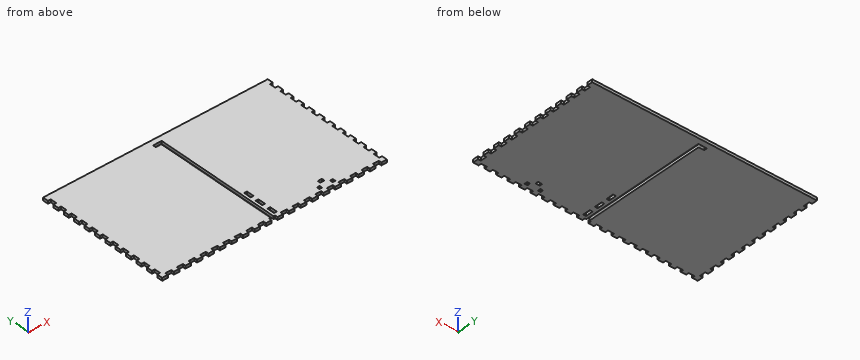
```python
from build123d import *

# Parameters (mm, degrees)
SKETCH1_W           = 508
SKETCH1_H           = 190.5
BOSS_EXTRUDE1_DEPTH = 6.35
SKETCH2_W           = 508
SKETCH2_H           = 190.5
SKETCH2_W_2         = 495.3
SKETCH2_H_2         = 177.8
BOSS_EXTRUDE2_DEPTH = 298.45
SKETCH3_W           = 6.35
SKETCH3_H           = 16.933333333
SKETCH3_H_2         = 16.933333334
CUT_EXTRUDE1_DEPTH  = 12.7
SKETCH4_W           = 6.35
SKETCH4_H           = 15.875
CUT_EXTRUDE2_DEPTH  = 6.35
SKETCH6_W           = 551.127140902
SKETCH6_H           = 227.623239157
CUT_EXTRUDE5_DEPTH  = 305.8
SKETCH5_W           = 13.368421053
SKETCH5_H           = 6.35
SKETCH5_W_2         = 13.368421052
CUT_EXTRUDE6_DEPTH  = 6.35
SKETCH7_W           = 6.35
SKETCH7_H           = 13.854545455
SKETCH7_H_2         = 13.854545454
CUT_EXTRUDE7_DEPTH  = 6.35
SKETCH8_W           = 9.652
SKETCH8_H           = 6.35
SKETCH8_W_2         = 6.35
LEVER_HOLE_DEPTH    = 7.35


with BuildPart() as part:
    # Sketch1 → Boss-Extrude1 (new body)
    with BuildSketch(Plane(origin=(0, 0, 0), x_dir=(1, 0, 0), z_dir=(0, 1, 0))):
        Rectangle(SKETCH1_W, SKETCH1_H)
    extrude(amount=BOSS_EXTRUDE1_DEPTH)

    # Sketch2 → Boss-Extrude2 (add)
    with BuildSketch(Plane(origin=(0, 6.35, 0), x_dir=(1, 0, 0), z_dir=(0, 1, 0))):
        Rectangle(SKETCH2_W, SKETCH2_H)
        Rectangle(SKETCH2_W_2, SKETCH2_H_2, mode=Mode.SUBTRACT)
    extrude(amount=BOSS_EXTRUDE2_DEPTH)

    # Sketch3 → Cut-Extrude1 (cut)
    with BuildSketch(Plane.XY.offset(95.25)):
        with BuildLine():
            Line((-3.302, 283.21), (-3.302, 6.35))
            Line((-3.302, 6.35), (3.302, 6.35))
            Line((3.302, 6.35), (3.302, 292.354))
            Line((3.302, 292.354), (-16.256, 292.354))
            Line((-16.256, 292.354), (-16.256, 285.75))
            Line((-16.256, 285.75), (-5.842, 285.75))
            ThreePointArc((-5.842, 285.75), (-4.045948776, 285.006051224), (-3.302, 283.21))
        make_face()
        with Locations((12.827, 80.433333334)):
            Rectangle(SKETCH3_W, SKETCH3_H)
        with Locations((12.827, 50.8)):
            Rectangle(SKETCH3_W, SKETCH3_H_2)
        with Locations((12.827, 21.166666667)):
            Rectangle(SKETCH3_W, SKETCH3_H)
    extrude(amount=-CUT_EXTRUDE1_DEPTH, mode=Mode.SUBTRACT)

    # Sketch4 → Cut-Extrude2 (cut)
    with BuildSketch(Plane.XY.offset(-88.9)):
        with Locations((-19.431, 284.1625)):
            Rectangle(SKETCH4_W, SKETCH4_H)
        with Locations((-19.431, 255.5875)):
            Rectangle(SKETCH4_W, SKETCH4_H)
        with Locations((-19.431, 227.0125)):
            Rectangle(SKETCH4_W, SKETCH4_H)
        with Locations((-19.431, 198.4375)):
            Rectangle(SKETCH4_W, SKETCH4_H)
        with Locations((-19.431, 169.8625)):
            Rectangle(SKETCH4_W, SKETCH4_H)
        with Locations((-19.431, 141.2875)):
            Rectangle(SKETCH4_W, SKETCH4_H)
        with Locations((-19.431, 112.7125)):
            Rectangle(SKETCH4_W, SKETCH4_H)
        with Locations((-19.431, 84.1375)):
            Rectangle(SKETCH4_W, SKETCH4_H)
        with Locations((-19.431, 55.5625)):
            Rectangle(SKETCH4_W, SKETCH4_H)
        with Locations((-19.431, 26.9875)):
            Rectangle(SKETCH4_W, SKETCH4_H)
    cut_extrude2 = extrude(amount=-CUT_EXTRUDE2_DEPTH, mode=Mode.SUBTRACT)

    # Mirror1: Cut-Extrude2 across plane
    add(cut_extrude2.mirror(Plane.ZY.offset(6.477)), mode=Mode.SUBTRACT)

    # Sketch6 → Cut-Extrude5 (cut, through all)
    with BuildSketch(Plane(origin=(0, 0, 0), x_dir=(1, 0, 0), z_dir=(0, 1, 0))):
        with Locations((15.161260543, 24.911619578)):
            Rectangle(SKETCH6_W, SKETCH6_H)
    extrude(amount=CUT_EXTRUDE5_DEPTH, mode=Mode.SUBTRACT)

    # Sketch5 → Cut-Extrude6 (cut)
    with BuildSketch(Plane(origin=(0, 0, 0), x_dir=(-1, 0, 0), z_dir=(0, -1, 0))):
        with Locations((-234.615789474, -92.075)):
            Rectangle(SKETCH5_W, SKETCH5_H)
        with Locations((-208.547368421, -92.075)):
            Rectangle(SKETCH5_W_2, SKETCH5_H)
        with Locations((-182.478947369, -92.075)):
            Rectangle(SKETCH5_W, SKETCH5_H)
        with Locations((-156.410526316, -92.075)):
            Rectangle(SKETCH5_W, SKETCH5_H)
        with Locations((-130.342105263, -92.075)):
            Rectangle(SKETCH5_W_2, SKETCH5_H)
        with Locations((-104.273684211, -92.075)):
            Rectangle(SKETCH5_W, SKETCH5_H)
        with Locations((-78.205263158, -92.075)):
            Rectangle(SKETCH5_W_2, SKETCH5_H)
        with Locations((-52.136842106, -92.075)):
            Rectangle(SKETCH5_W, SKETCH5_H)
        with Locations((-26.068421052, -92.075)):
            Rectangle(SKETCH5_W, SKETCH5_H)
        with Locations((0, -92.075)):
            Rectangle(SKETCH5_W_2, SKETCH5_H)
        with Locations((26.068421052, -92.075)):
            Rectangle(SKETCH5_W, SKETCH5_H)
        with Locations((52.136842106, -92.075)):
            Rectangle(SKETCH5_W, SKETCH5_H)
        with Locations((78.205263158, -92.075)):
            Rectangle(SKETCH5_W_2, SKETCH5_H)
        with Locations((104.273684211, -92.075)):
            Rectangle(SKETCH5_W, SKETCH5_H)
        with Locations((130.342105263, -92.075)):
            Rectangle(SKETCH5_W_2, SKETCH5_H)
        with Locations((156.410526316, -92.075)):
            Rectangle(SKETCH5_W, SKETCH5_H)
        with Locations((182.478947369, -92.075)):
            Rectangle(SKETCH5_W, SKETCH5_H)
        with Locations((208.547368421, -92.075)):
            Rectangle(SKETCH5_W_2, SKETCH5_H)
        with Locations((234.615789474, -92.075)):
            Rectangle(SKETCH5_W, SKETCH5_H)
    extrude(amount=-CUT_EXTRUDE6_DEPTH, mode=Mode.SUBTRACT)

    # Sketch7 → Cut-Extrude7 (cut)
    with BuildSketch(Plane(origin=(254, 0, 0), x_dir=(0, 0, -1), z_dir=(1, 0, 0))):
        with Locations((-92.075, 285.172727273)):
            Rectangle(SKETCH7_W, SKETCH7_H)
        with Locations((-92.075, 258.618181818)):
            Rectangle(SKETCH7_W, SKETCH7_H_2)
        with Locations((-92.075, 232.063636364)):
            Rectangle(SKETCH7_W, SKETCH7_H)
        with Locations((-92.075, 205.509090909)):
            Rectangle(SKETCH7_W, SKETCH7_H_2)
        with Locations((-92.075, 178.954545455)):
            Rectangle(SKETCH7_W, SKETCH7_H)
        with Locations((-92.075, 152.4)):
            Rectangle(SKETCH7_W, SKETCH7_H_2)
        with Locations((-92.075, 125.845454546)):
            Rectangle(SKETCH7_W, SKETCH7_H)
        with Locations((-92.075, 99.290909091)):
            Rectangle(SKETCH7_W, SKETCH7_H_2)
        with Locations((-92.075, 72.736363637)):
            Rectangle(SKETCH7_W, SKETCH7_H)
        with Locations((-92.075, 46.181818182)):
            Rectangle(SKETCH7_W, SKETCH7_H_2)
        with Locations((-92.075, 19.627272728)):
            Rectangle(SKETCH7_W, SKETCH7_H)
    cut_extrude7 = extrude(amount=-CUT_EXTRUDE7_DEPTH, mode=Mode.SUBTRACT)

    # Mirror2: Cut-Extrude7 across plane
    add(cut_extrude7.mirror(Plane(origin=(0, 0, 0), x_dir=(0, 0, 1), z_dir=(1, 0, 0))), mode=Mode.SUBTRACT)

    # Sketch8 → Lever Hole (cut, through all)
    with BuildSketch(Plane.XY.offset(95.25)):
        with Locations((130.342105263, 28.575)):
            Rectangle(SKETCH8_W, SKETCH8_H)
        with Locations((115.546605263, 15.875)):
            Rectangle(SKETCH8_W_2, SKETCH8_H)
        with Locations((145.137605263, 15.875)):
            Rectangle(SKETCH8_W_2, SKETCH8_H)
    extrude(amount=-LEVER_HOLE_DEPTH, mode=Mode.SUBTRACT)


solid = part.part
```
Geometry: final body of the model. Coordinates: model frame, mm. Round coordinates to 2 decimals unless told otherwise and drop trailing zeros. Write each loop counter-clockwise with the first axis right and the second up, starting at its lowest first coordinate (ties: lowest second). Pieces come first, ordered by that corner, then holes.
Item 1: Section query C-C (z = 93.25). Give the number of separate pieces and of enclosed holes in the cut face, plus the area to 3 significant figures.
Item 2: Material intervals for L1, parallel to X at y = 47, z = 90.25; L2, parallel to X at y = 88, z = 92.75; L3, parallel to X at y = 202, z = 92.5, sorted ascending.
Item 3: Section query B-B (x = 155). Return loops of the section in (y, z).
Item 4: Section query A-A (y = 180). Return loops of the section in (x, z), plus the area to 3 significant figures.
Item 5: Pin query (flat end, axial travel): P1, Ø1, axis at y = 101.5, z = 93, coming from the +X side. Return the tip coordinate at first contact, or that it passes through.
Completed:
1. separate pieces: 1
1. enclosed holes: 6
1. area: 149,000 mm2
2. L1: x = -247.65 to -3.3, 3.3 to 9.65, 16 to 247.65
2. L2: x = -254 to -3.3, 3.3 to 9.65, 16 to 254
2. L3: x = -247.65 to -3.3, 3.3 to 247.65
3. outline: (6.35, 88.9) - (304.8, 88.9) - (304.8, 95.25) - (6.35, 95.25) - close
4. outline: (-247.65, 88.9) - (-3.3, 88.9) - (-3.3, 95.25) - (-247.65, 95.25) - close; (3.3, 88.9) - (247.65, 88.9) - (247.65, 95.25) - (3.3, 95.25) - close
4. area: 3,100 mm2
5. P1: stops at x = 247.65
